Source: three-view drawing plus pictorial views. Frame: mm from the lowest corner of the part. Round coordinates to 2 decimals unless told otherwise and drop trailing zeros. Write each loop counter-clockwise with the first axis right and the second up, starting at its lowest first coordinate (ties: lowest second). Pieces come first, ordered by that corner, then holes. Notation, with made-up numbers: (-14.75, 39) - (30.25, 39) arc R20 cw to (30.25, 47) - close; hole circle Ø11 at (-25, 26). An arc over 180 degrees is marked (long way). Write each question's results on one line, items separated by ' | '.
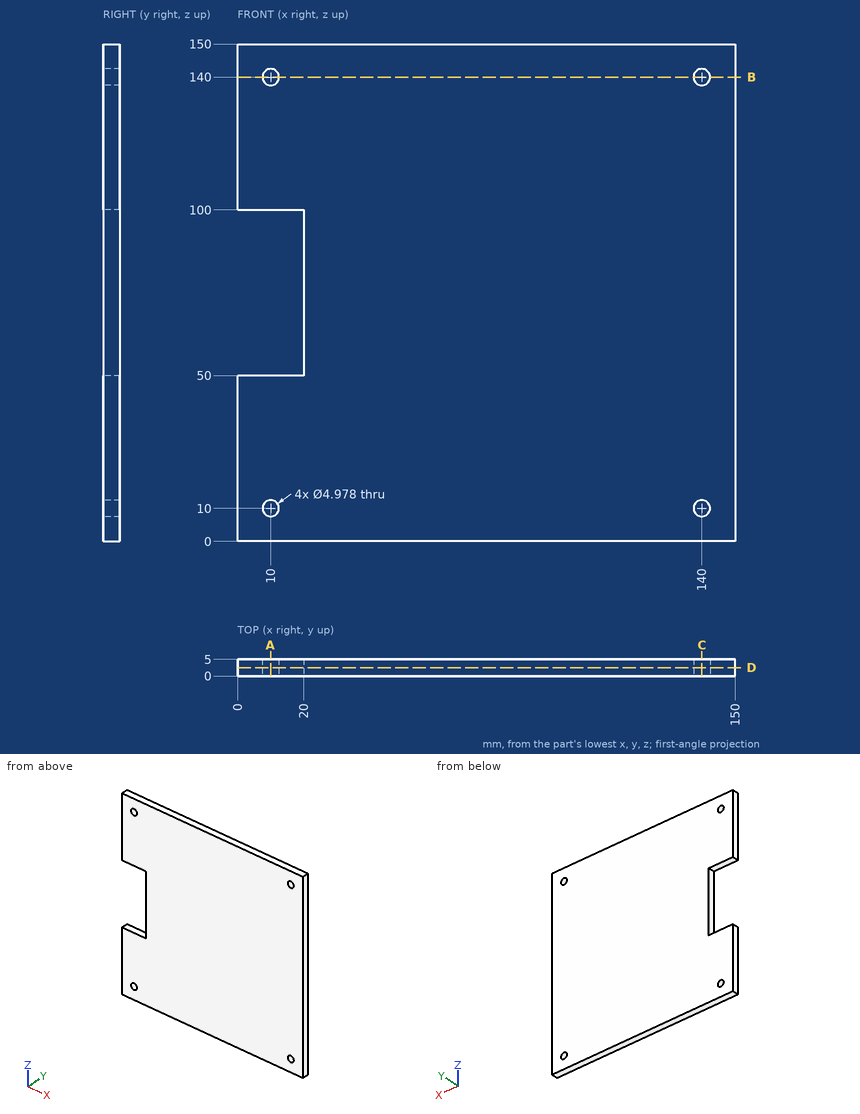
Q1. Section query C-C, the plane x = 140. Return loops of the section in (y, z).
Answer block:
outline: (0, 0) - (5, 0) - (5, 7.51) - (0, 7.51) - close; (0, 12.49) - (5, 12.49) - (5, 137.51) - (0, 137.51) - close; (0, 142.49) - (5, 142.49) - (5, 150) - (0, 150) - close
Q2. Section query D-D, the plane y = 2.55. Return loops of the section in (x, z), plus the area to 3 significant figures.
Answer block:
outline: (0, 0) - (150, 0) - (150, 150) - (0, 150) - (0, 100) - (20, 100) - (20, 50) - (0, 50) - close; hole circle Ø4.98 at (10, 10); hole circle Ø4.98 at (10, 140); hole circle Ø4.98 at (140, 10); hole circle Ø4.98 at (140, 140) | area: 21,400 mm2
Q3. Ray query, line 1 along X through (y, z) = (1.2, 10); line 2 along Z through (x, y) = (10, 2.3). Return the intervals inside material, ascending.
Answer block:
line 1: 0 to 7.51, 12.49 to 137.51, 142.49 to 150 | line 2: 0 to 7.51, 12.49 to 50, 100 to 137.51, 142.49 to 150
Q4. Pin query (flat end, axial travel): pin 1 (3 mm diameter, centred on y = 2.5, z = 57.5, fed in from -X). Return the tip coordinate at first contact, or that it passes through.
Answer block:
pin 1: x = 20
Q5. Section query B-B, the plane z = 140. Return loops of the section in (x, y).
Answer block:
outline: (0, 0) - (7.51, 0) - (7.51, 5) - (0, 5) - close; (12.49, 0) - (137.51, 0) - (137.51, 5) - (12.49, 5) - close; (142.49, 0) - (150, 0) - (150, 5) - (142.49, 5) - close
Q6. Section query A-A, the plane x = 10. Return loops of the section in (y, z).
Answer block:
outline: (0, 0) - (5, 0) - (5, 7.51) - (0, 7.51) - close; (0, 12.49) - (5, 12.49) - (5, 50) - (0, 50) - close; (0, 100) - (5, 100) - (5, 137.51) - (0, 137.51) - close; (0, 142.49) - (5, 142.49) - (5, 150) - (0, 150) - close
